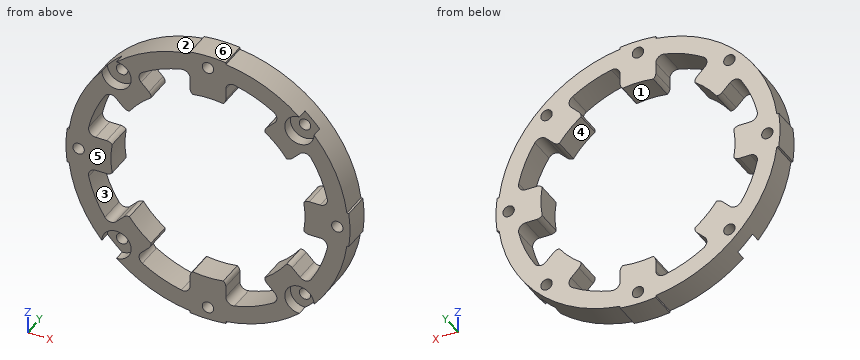
```python
from build123d import *

# Parameters (mm, degrees)
SKETCH1_R           = 1.6
BOSS_EXTRUDE1_DEPTH = 7.5
SKETCH3_R           = 27.2
CUT_EXTRUDE1_DEPTH  = 7.5
SKETCH4_R           = 4.1
CUT_EXTRUDE2_DEPTH  = 3


with BuildPart() as part:
    # Sketch1 → Boss-Extrude1 (new body)
    with BuildSketch(Plane(origin=(0, 0, 0), x_dir=(1, 0, 0), z_dir=(0, 1, 0))):
        with BuildLine():
            Line((-5, 38.930226046), (-5, 39.484680574))
            ThreePointArc((-5, 39.484680574), (0, 39.8), (5, 39.484680574))
            Line((5, 39.484680574), (5, 38.930226046))
            ThreePointArc((5, 38.930226046), (27.753941162, 27.753941162), (38.930226046, 5))
            Line((38.930226046, 5), (39.484680574, 5))
            ThreePointArc((39.484680574, 5), (39.8, 0), (39.484680574, -5))
            Line((39.484680574, -5), (38.930226046, -5))
            ThreePointArc((38.930226046, -5), (27.753941162, -27.753941162), (5, -38.930226046))
            Line((5, -38.930226046), (5, -39.484680574))
            ThreePointArc((5, -39.484680574), (0, -39.8), (-5, -39.484680574))
            Line((-5, -39.484680574), (-5, -38.930226046))
            ThreePointArc((-5, -38.930226046), (-27.753941162, -27.753941162), (-38.930226046, -5))
            Line((-38.930226046, -5), (-39.484680574, -5))
            ThreePointArc((-39.484680574, -5), (-39.8, 0), (-39.484680574, 5))
            Line((-39.484680574, 5), (-38.930226046, 5))
            ThreePointArc((-38.930226046, 5), (-27.753941162, 27.753941162), (-5, 38.930226046))
        make_face()
        with Locations(Location((36.25, 0, 0), (0, 0, 270))):
            Circle(SKETCH1_R, mode=Mode.SUBTRACT)
        with Locations(Location((25.632620818, -25.632620818, 0), (0, 0, 270))):
            Circle(SKETCH1_R, mode=Mode.SUBTRACT)
        with Locations(Location((0, -36.25, 0), (0, 0, 270))):
            Circle(SKETCH1_R, mode=Mode.SUBTRACT)
        with Locations(Location((-25.632620818, -25.632620818, 0), (0, 0, 270))):
            Circle(SKETCH1_R, mode=Mode.SUBTRACT)
        with Locations(Location((-36.25, 0, 0), (0, 0, 270))):
            Circle(SKETCH1_R, mode=Mode.SUBTRACT)
        with Locations(Location((-25.632620818, 25.632620818, 0), (0, 0, 270))):
            Circle(SKETCH1_R, mode=Mode.SUBTRACT)
        with Locations(Location((0, 36.25, 0), (0, 0, 270))):
            Circle(SKETCH1_R, mode=Mode.SUBTRACT)
        with Locations(Location((25.632620818, 25.632620818, 0), (0, 0, 270))):
            Circle(SKETCH1_R, mode=Mode.SUBTRACT)
        with BuildLine():
            Line((28.383070994, 5), (31.481145151, 5))
            ThreePointArc((31.481145151, 5), (33.041308132, 5.748644146), (33.43346423, 7.434108527))
            ThreePointArc((33.43346423, 7.434108527), (31.642873989, 13.106907559), (28.897737827, 18.384320724))
            ThreePointArc((28.897737827, 18.384320724), (27.428638298, 19.298827781), (25.796065122, 18.72499731))
            Line((25.796065122, 18.72499731), (23.605395877, 16.534328065))
            ThreePointArc((23.605395877, 16.534328065), (22.191182314, 15.948541627), (20.776968752, 16.534328065))
            Line((20.776968752, 16.534328065), (16.534328065, 20.776968752))
            ThreePointArc((16.534328065, 20.776968752), (15.948541627, 22.191182314), (16.534328065, 23.605395877))
            Line((16.534328065, 23.605395877), (18.72499731, 25.796065122))
            ThreePointArc((18.72499731, 25.796065122), (19.298827781, 27.428638298), (18.384320724, 28.897737827))
            ThreePointArc((18.384320724, 28.897737827), (13.106907559, 31.642873989), (7.434108527, 33.43346423))
            ThreePointArc((7.434108527, 33.43346423), (5.748644146, 33.041308132), (5, 31.481145151))
            Line((5, 31.481145151), (5, 28.383070994))
            ThreePointArc((5, 28.383070994), (4.414213562, 26.968857432), (3, 26.383070994))
            Line((3, 26.383070994), (-3, 26.383070994))
            ThreePointArc((-3, 26.383070994), (-4.414213562, 26.968857432), (-5, 28.383070994))
            Line((-5, 28.383070994), (-5, 31.481145151))
            ThreePointArc((-5, 31.481145151), (-5.748644146, 33.041308132), (-7.434108527, 33.43346423))
            ThreePointArc((-7.434108527, 33.43346423), (-13.106907559, 31.642873989), (-18.384320724, 28.897737827))
            ThreePointArc((-18.384320724, 28.897737827), (-19.298827781, 27.428638298), (-18.72499731, 25.796065122))
            Line((-18.72499731, 25.796065122), (-16.534328065, 23.605395877))
            ThreePointArc((-16.534328065, 23.605395877), (-15.948541627, 22.191182314), (-16.534328065, 20.776968752))
            Line((-16.534328065, 20.776968752), (-20.776968752, 16.534328065))
            ThreePointArc((-20.776968752, 16.534328065), (-22.191182314, 15.948541627), (-23.605395877, 16.534328065))
            Line((-23.605395877, 16.534328065), (-25.796065122, 18.72499731))
            ThreePointArc((-25.796065122, 18.72499731), (-27.428638298, 19.298827781), (-28.897737827, 18.384320724))
            ThreePointArc((-28.897737827, 18.384320724), (-31.642873989, 13.106907559), (-33.43346423, 7.434108527))
            ThreePointArc((-33.43346423, 7.434108527), (-33.041308132, 5.748644146), (-31.481145151, 5))
            Line((-31.481145151, 5), (-28.383070994, 5))
            ThreePointArc((-28.383070994, 5), (-26.968857432, 4.414213562), (-26.383070994, 3))
            Line((-26.383070994, 3), (-26.383070994, -3))
            ThreePointArc((-26.383070994, -3), (-26.968857432, -4.414213562), (-28.383070994, -5))
            Line((-28.383070994, -5), (-31.481145151, -5))
            ThreePointArc((-31.481145151, -5), (-33.041308132, -5.748644146), (-33.43346423, -7.434108527))
            ThreePointArc((-33.43346423, -7.434108527), (-31.642873989, -13.106907559), (-28.897737827, -18.384320724))
            ThreePointArc((-28.897737827, -18.384320724), (-27.428638298, -19.298827781), (-25.796065122, -18.72499731))
            Line((-25.796065122, -18.72499731), (-23.605395877, -16.534328065))
            ThreePointArc((-23.605395877, -16.534328065), (-22.191182314, -15.948541627), (-20.776968752, -16.534328065))
            Line((-20.776968752, -16.534328065), (-16.534328065, -20.776968752))
            ThreePointArc((-16.534328065, -20.776968752), (-15.948541627, -22.191182314), (-16.534328065, -23.605395877))
            Line((-16.534328065, -23.605395877), (-18.72499731, -25.796065122))
            ThreePointArc((-18.72499731, -25.796065122), (-19.298827781, -27.428638298), (-18.384320724, -28.897737827))
            ThreePointArc((-18.384320724, -28.897737827), (-13.106907559, -31.642873989), (-7.434108527, -33.43346423))
            ThreePointArc((-7.434108527, -33.43346423), (-5.748644146, -33.041308132), (-5, -31.481145151))
            Line((-5, -31.481145151), (-5, -28.383070994))
            ThreePointArc((-5, -28.383070994), (-4.414213562, -26.968857432), (-3, -26.383070994))
            Line((-3, -26.383070994), (3, -26.383070994))
            ThreePointArc((3, -26.383070994), (4.414213562, -26.968857432), (5, -28.383070994))
            Line((5, -28.383070994), (5, -31.481145151))
            ThreePointArc((5, -31.481145151), (5.748644146, -33.041308132), (7.434108527, -33.43346423))
            ThreePointArc((7.434108527, -33.43346423), (13.106907559, -31.642873989), (18.384320724, -28.897737827))
            ThreePointArc((18.384320724, -28.897737827), (19.298827781, -27.428638298), (18.72499731, -25.796065122))
            Line((18.72499731, -25.796065122), (16.534328065, -23.605395877))
            ThreePointArc((16.534328065, -23.605395877), (15.948541627, -22.191182314), (16.534328065, -20.776968752))
            Line((16.534328065, -20.776968752), (20.776968752, -16.534328065))
            ThreePointArc((20.776968752, -16.534328065), (22.191182314, -15.948541627), (23.605395877, -16.534328065))
            Line((23.605395877, -16.534328065), (25.796065122, -18.72499731))
            ThreePointArc((25.796065122, -18.72499731), (27.428638298, -19.298827781), (28.897737827, -18.384320724))
            ThreePointArc((28.897737827, -18.384320724), (31.642873989, -13.106907559), (33.43346423, -7.434108527))
            ThreePointArc((33.43346423, -7.434108527), (33.041308132, -5.748644146), (31.481145151, -5))
            Line((31.481145151, -5), (28.383070994, -5))
            ThreePointArc((28.383070994, -5), (26.968857432, -4.414213562), (26.383070994, -3))
            Line((26.383070994, -3), (26.383070994, 3))
            ThreePointArc((26.383070994, 3), (26.968857432, 4.414213562), (28.383070994, 5))
        make_face(mode=Mode.SUBTRACT)
    extrude(amount=BOSS_EXTRUDE1_DEPTH)

    # Sketch3 → Cut-Extrude1 (cut)
    with BuildSketch(Plane(origin=(0, 7.5, 0), x_dir=(1, 0, 0), z_dir=(0, 1, 0))):
        Circle(SKETCH3_R)
    extrude(amount=-CUT_EXTRUDE1_DEPTH, mode=Mode.SUBTRACT)

    # Sketch4 → Cut-Extrude2 (cut)
    with BuildSketch(Plane.XZ):
        with Locations((25.632620818, -25.632620818)):
            Circle(SKETCH4_R)
        with Locations((-25.632620818, -25.632620818)):
            Circle(SKETCH4_R)
        with Locations((-25.632620818, 25.632620818)):
            Circle(SKETCH4_R)
        with Locations((25.632620818, 25.632620818)):
            Circle(SKETCH4_R)
    extrude(amount=-CUT_EXTRUDE2_DEPTH, mode=Mode.SUBTRACT)


solid = part.part
```
Here's how the part is built. I have some questions about the finished solid (model axes, mm). Face numbers are marked on the shaded views. A direction names the side the tool comes from. Coordinates: 2 decimals unless noted, no trailing zeros. Order: outer loops, then holes, each group sorted by start corner. A loop starts at its lowest first (then second) coordinate and runs counter-clockwise, first axis right, second up.
1) Will these pins go through, and if not, where does the flat tip stop? pin 1 (5 mm diameter, centred on x = 25.63, z = 25.63, fed in from -Y); pin 2 (1 mm diameter, centred on x = -1.5, y = 4, fed in from +Z); pin 3 (10 mm diameter, centred on x = 26, z = 22, fed in from -Y); pin 4 (2.5 mm diameter, centred on x = -29, y = 4, fed in from +Z).
2) Which directions (+Z, -Z, +X, -X, +Y, -Y) give clear straight access to the entire face, cutting with the end or side of a thin tool? Please do the marked faces 1 and 2.
3) Imagine slicing it at C-C on z = -11. List the corners of the cut face in (x, y) for me.
4) Imagine slicing it at A-A on x = 0. List the corners of the cut face in (y, z) for me.
5) Imagine slicing it at D-D on x = 10. List the corners of the cut face in (y, z) for me, and give its area (3 significant figures).
6) Imagine slicing it at B-B on z = 0. List the corners of the cut face in (x, y) for me.
7) I need wall thicknesses on line 1 (X direction, y = 5.5, z = 0); line 2 (X direction, y = 6, z = -25); line 3 (X direction, y = 6.75, z = -28). Which ranges of each line are inside material? Lowest first, please.
8) We'd pull the mould along X, two halves only. Please class the marked faces 3, 4, 5 and 6: +X half, -X half, draft (parallel to the pull), parting line (faces both ways), or undercut.
Response values:
1. pin 1: stops at y = 3
1. pin 2: stops at z = 39.79
1. pin 3: stops at y = 0
1. pin 4: stops at z = 27.76
2. face 1: +Y, -Y
2. face 2: +Z, -X, +Y, -Y
3. outline: (-37.68, 0) - (-32.44, 0) - (-32.44, 7.5) - (-37.68, 7.5) - close; (32.44, 0) - (37.68, 0) - (37.68, 7.5) - (32.44, 7.5) - close
4. outline: (0, -39.8) - (7.5, -39.8) - (7.5, -37.85) - (0, -37.85) - close; (0, -34.65) - (7.5, -34.65) - (7.5, -27.2) - (0, -27.2) - close; (0, 27.2) - (7.5, 27.2) - (7.5, 34.65) - (0, 34.65) - close; (0, 37.85) - (7.5, 37.85) - (7.5, 39.8) - (0, 39.8) - close
5. outline: (0, -37.95) - (7.5, -37.95) - (7.5, -32.76) - (0, -32.76) - close; (0, 32.76) - (7.5, 32.76) - (7.5, 37.95) - (0, 37.95) - close
5. area: 78.0 mm2
6. outline: (-39.8, 0) - (-37.85, 0) - (-37.85, 7.5) - (-39.8, 7.5) - close; (-34.65, 0) - (-27.2, 0) - (-27.2, 7.5) - (-34.65, 7.5) - close; (27.2, 0) - (34.65, 0) - (34.65, 7.5) - (27.2, 7.5) - close; (37.85, 0) - (39.8, 0) - (39.8, 7.5) - (37.85, 7.5) - close
7. line 1: x = -39.8 to -37.85, -34.65 to -27.2, 27.2 to 34.65, 37.85 to 39.8
7. line 2: x = -30.26 to -27.1, -24.16 to -17.93, 17.93 to 24.16, 27.1 to 30.26
7. line 3: x = -27.51 to -19.15, -4.96 to 4.96, 19.15 to 27.51
8. face 3: undercut
8. face 4: undercut
8. face 5: draft
8. face 6: parting line
